The drawing under review shows one solid part. Ordinate dimensions are in mm from its lowest x, y, z. A direction names the side the tool comes from. Coordinates: 2 decimals unless noted, no trailing zeros. Order: outer loops, then holes, each group sorted by start corner. A loop starts at its lowest first (then second) coordinate and runs counter-clockwise, first axis right, second up.
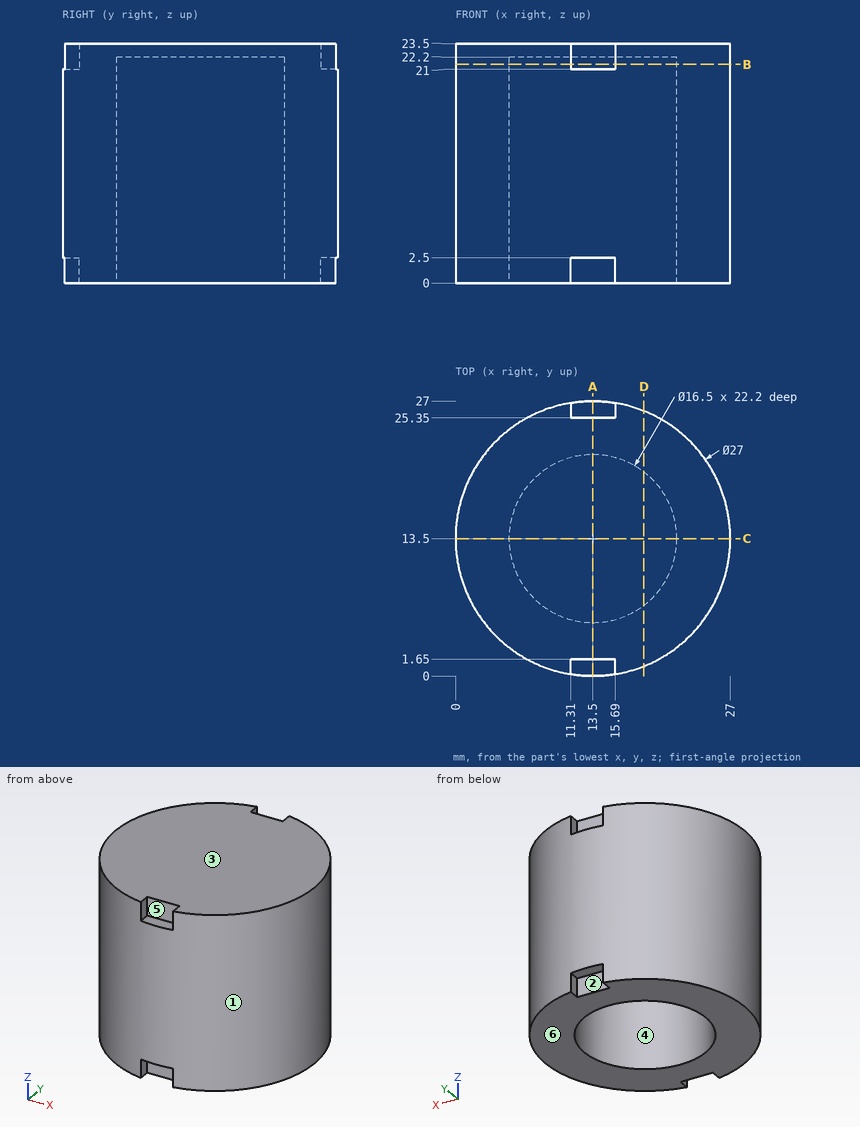
1. Clearance check with flat-ended pins moving along their axes: pin 1 Ø1.6 at (y, z) = (1, 21.5) entering from -X (1 decimal); pin 2 Ø0.7 at (y, z) = (1, 2) entering from +X (1 decimal); pin 3 Ø0.8 at (x, y) = (13, 1) entering from -Z. State where each tip first meets the part, or that it passes through.
Answer below:
pin 1: stops at x = 6.8
pin 2: stops at x = 19.4
pin 3: stops at z = 2.5
2. Take a section at D-D, the plane x = 18.5. Give the boundary of the cut face in (y, z), plus the area to 3 significant figures.
Answer below:
outline: (0.96, 0) - (6.94, 0) - (6.94, 22.2) - (20.06, 22.2) - (20.06, 0) - (26.04, 0) - (26.04, 23.5) - (0.96, 23.5) - close
area: 298 mm2
3. Machinability: for the marked faces 4, 5 and 6, which of the approach directions +Z, -Z, +X, -X, +Y, -Y give a long, thin tool a straight path to every point of the face, cutting with its end or side? Answer none if there is none.
Answer below:
face 4: -Z
face 5: +Z, -Y
face 6: -Z, +X, -X, +Y, -Y
4. Take a section at A-A, the plane x = 13.5. Give the boundary of the cut face in (y, z).
Answer below:
outline: (0, 2.5) - (1.65, 2.5) - (1.65, 0) - (5.25, 0) - (5.25, 22.2) - (21.75, 22.2) - (21.75, 0) - (25.35, 0) - (25.35, 2.5) - (27, 2.5) - (27, 21) - (25.35, 21) - (25.35, 23.5) - (1.65, 23.5) - (1.65, 21) - (0, 21) - close
5. Take a section at B-B, the plane z = 21.5. Give the boundary of the cut face in (x, y), plus the area to 3 significant figures.
Answer below:
outline: (11.31, 0.18) - (11.31, 1.65) - (15.69, 1.65) - (15.69, 0.18) arc R13.5 ccw to (15.69, 26.82) - (15.69, 25.35) - (11.31, 25.35) - (11.31, 26.82) arc R13.5 ccw to start; hole circle Ø16.5 at (13.5, 13.5)
area: 345 mm2
6. Take a section at C-C, the plane y = 13.5. Give the boundary of the cut face in (x, z), plus the area to 3 significant figures.
Answer below:
outline: (0, 0) - (5.25, 0) - (5.25, 22.2) - (21.75, 22.2) - (21.75, 0) - (27, 0) - (27, 23.5) - (0, 23.5) - close
area: 268 mm2
7. The part is to be moulded in two halves that separate along X. For the marked faces 1, 2 and 3, say which applies: +X half, -X half, draft (parallel to the pull), parting line (faces both ways), or undercut.
Answer below:
face 1: parting line
face 2: undercut
face 3: draft
8. To check wall thickness, follow L1, parallel to Y at x = 13.5, z = 17; L2, parallel to X at y = 12, z = 21.75; L3, parallel to Z at x = 8.75, y = 13.25. State the ranges of each line that lie inside material, in increasing order.
Answer below:
L1: y = 0 to 5.25, 21.75 to 27
L2: x = 0.08 to 5.39, 21.61 to 26.92
L3: z = 22.2 to 23.5
